Autodesk Inventor part; units mm, degrees
ref_plane "YZ Plane" through (0, 0, 0) normal (1, 0, 0) x (0, 1, 0)
ref_plane "XZ Plane" through (0, 0, 0) normal (0, 1, 0) x (-1, 0, 0)
ref_plane "XY Plane" through (0, 0, 0) normal (0, 0, 1) x (1, 0, 0)
sketch "Sketch1" plane through (0, 0, 0) normal (0, 0, 1) x (1, 0, 0)
  point P0 (0, 0)
sketch "Sketch2" plane through (0, 0, 0) normal (0, 0, 1) x (1, 0, 0)
  circle A0 centre (0, 0) radius 18.4
  dimension "d0" = 36.8
extrude "Extrusion1" add sketch "Sketch2" against normal blind 21.5
sketch "Sketch3" plane through (0, 0, -21.5) normal (0, 0, -1) x (-1, 0, 0)
  circle A0 centre (0, 0) radius 17.4
  dimension "d3" = 34.8
extrude "Extrusion2" add sketch "Sketch3" along normal blind 30.7
sketch "Sketch4" plane through (0, 0, -52.2) normal (0, 0, -1) x (-1, 0, 0)
  circle A0 centre (0, 0) radius 17
  dimension "d6" = 34
extrude "Extrusion3" add sketch "Sketch4" along normal blind 15.4
sketch "Sketch5" plane through (0, 0, 0) normal (0, 0, 1) x (1, 0, 0)
  circle A0 centre (-15.5, 0) radius 1.5
  circle A1 centre (0, 0) radius 18.4
  line L0 (-18.4, 0) -> (18.4, 0)
  line L1 (-1.5961, -18.3306) -> (-1.5961, -18.3306)
  line L2 (0, 18.4) -> (0, -18.4)
  circle A2 centre (0, -7) radius 6
  circle A3 centre (15.5, 0) radius 1.5
  circle A4 centre (0, 0) radius 15.5
  line L3 (-11.863, 20.6629) -> (9.25, -15.9059)
  circle A5 centre (0, 0) radius 18.4
  line L4 (-9.2, -15.9349) -> (9.2, 15.9349)
  circle A6 centre (7.8, -13.3944) radius 1.5
  circle A7 centre (7.75, 13.4234) radius 1.5
  circle A8 centre (-7.75, -13.4234) radius 1.5
  circle A9 centre (-7.6999, 13.4522) radius 1.5
  point P0 (7.75, 13.4234)
  point P1 (7.8, -13.3944)
  dimension "d10" = 3
  dimension "d11" = 12
  dimension "d12" = 7
  dimension "d15" = 3
  dimension "d16" = 31
  dimension "d17" = 2.9
  dimension "d19" = 60
  dimension "d20" = 60
  dimension "d21" = 3
  dimension "d22" = 3
  dimension "d23" = 3
  dimension "d24" = 3
extrude "Extrusion4" add sketch "Sketch5" along normal blind 6 contours A2 L3 L2 | L2 A2 L4 | L4 A2 | A2 L3 picked at (-1.9225, -8.5027)
extrude "Extrusion5" cut sketch "Sketch5" against normal blind 3 contours L0 A4 A0 | A0 A4 L0 | A4 L0 A0 | A0 L0 A4 | A9 L3 A4 | A4 L3 A9 | A8 L4 A4 | A4 L4 A8 | L3 A9 A4 | A4 A9 L3 | L4 A8 A4 | A4 A8 L4 | A3 A4 L0 | L0 A4 A3 | A7 A4 L4 | L4 A4 A7 | A4 A3 L0 | L0 A3 A4 | A7 L4 A4 | L4 A7 A4 | A6 L3 A4 | A4 L3 A6 | L3 A4 A6 | A4 L3 A6
sketch "Sketch6" plane through (0, -7, 6) normal (0, 0, 1) x (1, 0, 0)
  circle A0 centre (0, 0) radius 6
  circle A1 centre (0, 0) radius 3
  point P0 (0, 7)
  dimension "d27" = 6
extrude "Extrusion6" add sketch "Sketch6" along normal blind 16 contours A1
sketch "Sketch7" plane through (0, -7, 22) normal (0, 0, 1) x (1, 0, 0)
  line L0 (-6, 3) -> (6, 3)
  line L1 (6, 3) -> (6, 2.4)
  line L2 (6, 2.4) -> (-6, 2.4)
  line L3 (-6, 2.4) -> (-6, 3)
  circle A0 centre (0, 0) radius 6
  circle A1 centre (0, 0) radius 3
  circle A2 centre (0, 0) radius 3
  line L4 (0, 3) -> (0, -3)
  point P0 (0, 7)
  dimension "d30" = 0.6
extrude "Extrusion7" cut sketch "Sketch7" against normal up to surface (16 mm away) contours L0 A0 L2 L3 | L0 A1 L2 A0 | L0 A0 L2 A1 | L4 L2 A1 | A1 L2 L4 | L0 L1 L2 A0 picked at (-1.016, 2.5094) picked at (1.016, 2.5094)
properties part number "Motor"
CAD build for the part. Positions are in the model's coordinates, mm. A direction names the side the tool comes from. Coordinates: 2 decimals unless noted, no trailing zeros. Order: outer loops, then holes, each group sorted by start corner. A loop starts at its lowest first (then second) coordinate and runs counter-clockwise, first axis right, second up. Notation, with made-up numbers: (32.25, 77.25) - (85.25, 77.25) arc R19 cw to (85.25, 100.25) - close; hole circle Ø3 at (16.5, 13). An arc over 180 degrees is marked (long way). Use a Markdown table: item, result. Add a question column.
(1) Pull direction X, two halves, no side cores. Call faces 1 (the face through (0, -4, 6)), 2 (the face through (14, 0, -1)), 3 (the face through (-14.6, -11.2, -10.6)), 4 (the face through (6.644, 14.437, -1.479)): +X half, -X half, draft (parallel to the pull), parting line (faces both ways), or undercut.
(2) Drill centre lines: line 1 along Z through (x, y) = (-8, 11); line 2 along Z through (x, y) = (-14, -11); line 3 along Y through (x, z) = (15, -1). Where is each one in solid material? Low to high. Write a range as [from, to].
(3) Saw through at D-D (x = -4). Give the cut face in (y, z).
(4) Saw through at A-A (x = 0). Give the cut face in (y, z), then the cut area to 3 significant figures.
(5) Saw through at C-C (z = -16). Give the cut face in (x, y).
(6) Flat gauge pins, fed straight in: pin 1 (2 mm diameter, centred on x = -10.5, y = -3.5, fed in from +Z); pin 2 (1.5 mm diameter, centred on x = -15, y = 0.5, fed in from +Z); pin 3 (1.5 mm diameter, centred on x = -9, z = -50.5, fed in from -Y). Where does each tip first touch, or does it go through?
(7) Saw through at B-B (y = 0). Give the cut face in (x, z).
(8) Which spindle directions (+Z, -Z, +X, -X, +Y, -Y) get a long thin tool onto all of the face, cutting with end or side? Do faces 5 (the face through (0, -4.6, 14)), 6 (the face through (15, 0, -3)), 7 (the face through (-9.139, -14.334, -59.792)). Say none if no direction does.
Solved:
| question | item | result |
|---|---|---|
| 1 | face 1 | draft |
| 1 | face 2 | undercut |
| 1 | face 3 | parting line |
| 1 | face 4 | undercut |
| 2 | line 1 | z = [-67.6, 0] |
| 2 | line 2 | z = [-21.5, 0] |
| 2 | line 3 | y = [-10.66, -1.41], [1.41, 10.66] |
| 3 | outline | (-17.96, -21.5) - (-16.93, -21.5) - (-16.93, -52.2) - (-16.52, -52.2) - (-16.52, -67.6) - (16.52, -67.6) - (16.52, -52.2) - (16.93, -52.2) - (16.93, -21.5) - (17.96, -21.5) - (17.96, 0) - (-2.53, 0) - (-2.53, 6) - (-11.47, 6) - (-11.47, 0) - (-17.96, 0) - close |
| 4 | outline | (-18.4, -21.5) - (-17.4, -21.5) - (-17.4, -52.2) - (-17, -52.2) - (-17, -67.6) - (17, -67.6) - (17, -52.2) - (17.4, -52.2) - (17.4, -21.5) - (18.4, -21.5) - (18.4, 0) - (-1, 0) - (-1, 6) - (-4.6, 6) - (-4.6, 22) - (-10, 22) - (-10, 6) - (-13, 6) - (-13, 0) - (-18.4, 0) - close |
| 4 | area | 2,540 mm² |
| 5 | outline | circle Ø36.8 at (0, 0) |
| 6 | pin 1 | stops at z = 0 |
| 6 | pin 2 | stops at z = -3 |
| 6 | pin 3 | stops at y = -15.32 |
| 7 | outline | (-18.4, -21.5) - (-17.4, -21.5) - (-17.4, -52.2) - (-17, -52.2) - (-17, -67.6) - (17, -67.6) - (17, -52.2) - (17.4, -52.2) - (17.4, -21.5) - (18.4, -21.5) - (18.4, 0) - (17, 0) - (17, -3) - (14, -3) - (14, 0) - (-14, 0) - (-14, -3) - (-17, -3) - (-17, 0) - (-18.4, 0) - close |
| 8 | face 5 | +Z, +X, -X, +Y |
| 8 | face 6 | +Z |
| 8 | face 7 | -Z |
